Work out the finished part from the listing and answer in its coordinate system (mm). A direction names the side the tool comes from. Round coordinates to 2 decimals unless told otherwise and drop trailing zeros. Order: outer loops, then holes, each group sorted by start corner. A loop starts at its lowest first (then second) coordinate and runs counter-clockwise, first axis right, second up. Notation, with made-up numbers: (80, -7) - (127, -7) arc R21 ccw to (127, 15) - close; hole circle Ø9 at (88.5, -30.75). An arc over 180 degrees is marked (long way). Put each result on its own line as item: value.
```python
from build123d import *
from OCP.BRepFilletAPI import BRepFilletAPI_MakeChamfer

# Parameters (mm, degrees)
SKETCH2_R               = 2.75
SKETCH2_R_2             = 9.733125881
BOSS_EXTRUDE1_DEPTH     = 8
CHAMFER1_SIZE           = 2
BOSS_EXTRUDE3_DEPTH     = 12
CHAMFER2_SIZE           = 2
CUT_EXTRUDE2_DEPTH      = 82.236487908
CUT_EXTRUDE2_DEPTH_BACK = 82.236487908
CHAMFER3_SIZE           = 1
CHAMFER3_SIZE_2         = 1.020612224


with BuildPart() as part:
    # Sketch2 → Boss-Extrude1 (new body)
    with BuildSketch(Plane(origin=(0, 0, 0), x_dir=(1, 0, 0), z_dir=(0, 1, 0))):
        with BuildLine():
            Line((58.828710372, -43.095584491), (65.546224794, -36.37807007))
            Line((65.546224794, -36.37807007), (37.261953546, -8.093798822))
            ThreePointArc((37.261953546, -8.093798822), (-0.530330086, 16.263455967), (23.826924704, -21.528827665))
            Line((23.826924704, -21.528827665), (52.111195951, -49.813098912))
            Line((52.111195951, -49.813098912), (58.828710372, -43.095584491))
        make_face()
        with Locations(Location((0, 0, 0), (0, 0, 270))):
            Circle(SKETCH2_R, mode=Mode.SUBTRACT)
        with Locations(Location((31.466251763, 0, 0), (0, 0, 270))):
            Circle(SKETCH2_R, mode=Mode.SUBTRACT)
        with Locations(Location((15.733125881, 15.733125881, 0), (0, 0, 270))):
            Circle(SKETCH2_R, mode=Mode.SUBTRACT)
        with Locations(Location((15.733125881, -15.733125881, 0), (0, 0, 270))):
            Circle(SKETCH2_R, mode=Mode.SUBTRACT)
        with Locations(Location((4.608125881, 11.125, 0), (0, 0, 270))):
            Circle(SKETCH2_R, mode=Mode.SUBTRACT)
        with Locations(Location((15.733125881, 0, 0), (0, 0, 270))):
            Circle(SKETCH2_R_2, mode=Mode.SUBTRACT)
    extrude(amount=BOSS_EXTRUDE1_DEPTH)

    # Chamfer1
    chamfer1_edges = [part.edges().sort_by_distance(p)[0] for p in [
        (65.546224794, 4, 36.37807007),
        (52.111195951, 4, 49.813098912),
    ]]
    chamfer(chamfer1_edges, length=CHAMFER1_SIZE)

    # Sketch7 → Boss-Extrude3 (add)
    with BuildSketch(Plane(origin=(0, 0, 0), x_dir=(-1, 0, 0), z_dir=(0, -1, 0))):
        Polygon((-53.525409514, -48.39888535), (-64.132011231, -37.792283632), (-64.132011231, -34.963856507), (-56.016040068, -26.847885344), (-42.581011226, -40.282914187), (-50.696982389, -48.39888535), align=None)
    extrude(amount=BOSS_EXTRUDE3_DEPTH)

    # Sketch8 → Cut-Revolve2 (revolve, cut)
    with BuildSketch(Plane(origin=(47.426613526, 0, 47.426613526), x_dir=(0.7071067811865475, 0, -0.7071067811865477), z_dir=(0.7071067811865477, 0, 0.7071067811865475)), mode=Mode.PRIVATE) as cut_revolve2_sk:
        Polygon((5.525, -12), (5.125, 8), (7.625, 8), (7.625, -12), align=None)
    revolve(cut_revolve2_sk.sketch.rotate(Axis((52.818302732, 8, 42.034924319), (0, -1, 0)), 315), axis=Axis((52.818302732, 8, 42.034924319), (0, -1, 0)), mode=Mode.SUBTRACT)

    # Sketch9 → Cut-Revolve3 (revolve, cut)
    with BuildSketch(Plane(origin=(47.426613526, 0, 47.426613526), x_dir=(0.7071067811865475, 0, -0.7071067811865477), z_dir=(0.7071067811865477, 0, 0.7071067811865475)), mode=Mode.PRIVATE) as cut_revolve3_sk:
        Polygon((14.625, -12), (16.725, -12), (17.125, 8), (14.625, 8), align=None)
    revolve(cut_revolve3_sk.sketch.rotate(Axis((57.768050201, 8, 37.085176851), (0, -1, 0)), 135), axis=Axis((57.768050201, 8, 37.085176851), (0, -1, 0)), mode=Mode.SUBTRACT)

    # Chamfer2
    chamfer2_edges = [part.edges().sort_by_distance(p)[0] for p in [
        (49.298525647, 0, 33.565399766),
    ]]
    chamfer(chamfer2_edges, length=CHAMFER2_SIZE)

    # Sketch10 → Cut-Extrude2 (cut, two sides: drawn at the far end of the back side and taken through both)
    with BuildSketch(Plane.XZ.offset(-CUT_EXTRUDE2_DEPTH_BACK)):
        with BuildLine():
            Line((29.768176219, 16.863477462), (42.110295184, 29.205596427))
            ThreePointArc((42.110295184, 29.205596427), (44.966986546, 29.176755666), (44.880476019, 26.321228875))
            Line((44.880476019, 26.321228875), (32.827718409, 14.312209061))
            ThreePointArc((32.827718409, 14.312209061), (29.901532194, 13.913228795), (29.768176219, 16.863477462))
        make_face()
    extrude(amount=CUT_EXTRUDE2_DEPTH + CUT_EXTRUDE2_DEPTH_BACK, mode=Mode.SUBTRACT)

    # Chamfer3
    chamfer3_edges_1 = [part.edges().sort_by_distance(p)[0] for p in [
        (52.818302732, 8, 39.534924319),
    ]]
    chamfer3_side_1 = [part.faces().sort_by_distance(p)[0] for p in [
        (52.818302732, 8, 39.514924319),
    ]]
    chamfer3_edges_2 = [part.edges().sort_by_distance(p)[0] for p in [
        (57.768050201, 8, 34.585176851),
    ]]
    chamfer3_side_2 = [part.faces().sort_by_distance(p)[0] for p in [
        (57.768050201, 8, 34.565176851),
    ]]
    chamfer3 = BRepFilletAPI_MakeChamfer(part.part.solid().wrapped)
    for e in chamfer3_edges_1:
        chamfer3.Add(CHAMFER3_SIZE - 0.0001, CHAMFER3_SIZE_2 - 0.0001, e.wrapped, chamfer3_side_1[0].wrapped)
    for e in chamfer3_edges_2:
        chamfer3.Add(CHAMFER3_SIZE - 0.0001, CHAMFER3_SIZE_2 - 0.0001, e.wrapped, chamfer3_side_2[0].wrapped)
    add(Compound.cast(chamfer3.Shape()), mode=Mode.REPLACE)  # a hair under: the kernel refuses the full size


solid = part.part
```
1) A cutting plane is placed at A-A on z = 0. Write down the section's boundary in (x, y), then the cut area to 3 significant figures.
Findings below:
outline: (-7.27, 0) - (-2.75, 0) - (-2.75, 8) - (-7.27, 8) - close; (2.75, 0) - (6, 0) - (6, 8) - (2.75, 8) - close; (25.47, 0) - (28.72, 0) - (28.72, 8) - (25.47, 8) - close; (34.22, 0) - (38.73, 0) - (38.73, 8) - (34.22, 8) - close
area: 124 mm2
2) Straight lines are drawn through the part: L1, parallel to X at y = 3, z = 0; L2, parallel to X at y = 6.75, z = 15; L3, parallel to X at y = 2, z = 24. For each, find the intervals that lie inside material, in ascending order. Write a range as from..to.
Findings below:
L1: x = -7.27..-2.75, 2.75..6, 25.47..28.72, 34.22..38.73
L2: x = -1.7..13.08, 18.38..29.23, 33.52..44.17
L3: x = 26.3..36.9, 42.55..53.17
3) A cutting plane is placed at C-C on z = 24.5. Write down the section's boundary in (x, y), then the cut area to 3 significant figures.
Findings below:
outline: (26.8, 0) - (37.4, 0) - (37.4, 8) - (26.8, 8) - close; (43.05, 0) - (53.67, 0) - (53.67, 8) - (43.05, 8) - close
area: 170 mm2
4) Given pin 1 Ø18.5 at (x, z) = (25.5, 21) entering from -Y; pin 2 Ø6.5 at (x, z) = (15.73, -15.73) entering from +Y; pin 3 Ø4.5 at (x, z) = (0, 0) entering from +Y; pin 4 Ø12 at (y, z) = (2.5, 13) entering from -X, each flat-ended and moving along its own axis, determine where each tip first touches the part or whether it passes through.
Findings below:
pin 1: stops at y = 0
pin 2: stops at y = 8
pin 3: passes through
pin 4: stops at x = -6.18
5) For a pull along X with two mould halves and no side action, classify faces 1 (the flat face through (23, 0, 8)), 2 (the flat face through (49.393, -6.93, 33.471)), 3 (the flat face through (35.853, 4.056, 22.948)) as pulls with the +X half, pulls with the -X half, needs draft (parallel to the pull), parting line crosses it, or undercut.
Findings below:
face 1: needs draft
face 2: pulls with the -X half
face 3: undercut
6) A cutting plane is placed at B-B on y = 4.5. Give the number of separate pieces and of enclosed holes in the cut face, then the cut area to 3 significant figures.
Findings below:
separate pieces: 1
enclosed holes: 9
area: 1,860 mm2
7) For faces 4 (the flat face through (52, -2, 48.399)), 5 (the flat face through (38.94, 4.06, 20.4)), 6 (the conical face through (54.213, -2.377, 40.216)), determine the directions among +Z, -Z, +X, -X, +Y, -Y from which every point of the face is accessible in a straight line to the end or side of a thin tool.
Findings below:
face 4: +Z, +X, -X, +Y, -Y
face 5: +Y, -Y
face 6: +Y
8) A cutting plane is placed at D-D on x = 14. Write down the section's boundary in (y, z).
Findings below:
outline: (0, -22.93) - (8, -22.93) - (8, -17.87) - (0, -17.87) - close; (0, -13.6) - (8, -13.6) - (8, -9.58) - (0, -9.58) - close; (0, 9.58) - (8, 9.58) - (8, 13.6) - (0, 13.6) - close; (0, 17.87) - (8, 17.87) - (8, 22.93) - (0, 22.93) - close
